Read the model definition and answer for the solid it produces. Units are mm, in the model's axes. Face numbers are marked on the shaded views. A direction names the side the tool comes from. Coordinates: 2 decimals unless noted, no trailing zeros. Loops run counter-clockwise (first coordinate to the right, second up) from the corner with the lowest first, then second, coordinate; pieces in that order, holes last.
from build123d import *

# Parameters (mm, degrees)
CROQUIS1_R              = 1.625
SALIENTE_EXTRUIR1_DEPTH = 3
CORTAR_EXTRUIR1_DEPTH   = 2
CROQUIS4_W              = 29.5
CROQUIS4_H              = 10.2
SALIENTE_EXTRUIR2_DEPTH = 3
SALIENTE_EXTRUIR3_DEPTH = 3
CROQUIS7_W              = 10
CROQUIS7_H              = 3
SALIENTE_EXTRUIR4_DEPTH = 5
CROQUIS9_W              = 10
CROQUIS9_H              = 3
SALIENTE_EXTRUIR5_DEPTH = 10
CROQUIS10_R             = 1.625
CORTAR_EXTRUIR2_DEPTH   = 3
CORTAR_EXTRUIR3_DEPTH   = 2


with BuildPart() as part:
    # Croquis1 → Saliente-Extruir1 (new body)
    with BuildSketch(Plane.XY):
        Polygon((-40.458841365, -24.7), (-77.458841365, -24.7), (-77.458841365, -14.45), (-47.958841365, -14.45), (-47.958841365, -17.2), (-40.458841365, -17.2), align=None)
        with Locations((-44.208841365, -20.95)):
            Circle(CROQUIS1_R, mode=Mode.SUBTRACT)
    extrude(amount=SALIENTE_EXTRUIR1_DEPTH)

    # Croquis2 → Cortar-Extruir1 (cut)
    with BuildSketch(Plane.XY.offset(3)):
        Polygon((-44.232492922, -17.739034302), (-46.977793452, -19.324034302), (-46.977793452, -22.494034302), (-44.232492922, -24.079034302), (-41.487192392, -22.494034302), (-41.487192392, -19.324034302), align=None)
    extrude(amount=-CORTAR_EXTRUIR1_DEPTH, mode=Mode.SUBTRACT)

    # Croquis4 → Saliente-Extruir2 (add)
    with BuildSketch(Plane(origin=(0, -14.45, 0), x_dir=(1, 0, 0), z_dir=(0, 1, 0))):
        with Locations((-62.708841365, 2.1)):
            Rectangle(CROQUIS4_W, CROQUIS4_H)
    extrude(amount=SALIENTE_EXTRUIR2_DEPTH)

    # Croquis6 → Saliente-Extruir3 (add)
    with BuildSketch(Plane.XY.offset(3)):
        Polygon((-62.708841365, -11.45), (-67.708841365, -11.45), (-67.708841365, -5), (-57.708841365, -5), (-57.708841365, -11.45), align=None)
    extrude(amount=-SALIENTE_EXTRUIR3_DEPTH)

    # Croquis7 → Saliente-Extruir4 (add)
    with BuildSketch(Plane(origin=(0, -5, 0), x_dir=(1, 0, 0), z_dir=(0, 1, 0))):
        with Locations((-62.708841365, -1.5)):
            Rectangle(CROQUIS7_W, CROQUIS7_H)
    extrude(amount=SALIENTE_EXTRUIR4_DEPTH)

    # Croquis9 → Saliente-Extruir5 (add)
    with BuildSketch(Plane.XY.offset(3)):
        with Locations((-62.708841365, -6.5)):
            Rectangle(CROQUIS9_W, CROQUIS9_H)
    extrude(amount=SALIENTE_EXTRUIR5_DEPTH)

    # Croquis10 → Cortar-Extruir2 (cut)
    with BuildSketch(Plane.XZ.offset(8)):
        with Locations(Location((-62.708841365, 8, 0), (0, 0, 270))):
            Circle(CROQUIS10_R)
    extrude(amount=-CORTAR_EXTRUIR2_DEPTH, mode=Mode.SUBTRACT)

    # Croquis11 → Cortar-Extruir3 (cut)
    with BuildSketch(Plane.XZ.offset(8)):
        Polygon((-62.708841365, 4.83), (-59.963540835, 6.415), (-59.963540835, 9.585), (-62.708841365, 11.17), (-65.454141895, 9.585), (-65.454141895, 6.415), align=None)
    extrude(amount=-CORTAR_EXTRUIR3_DEPTH, mode=Mode.SUBTRACT)


solid = part.part
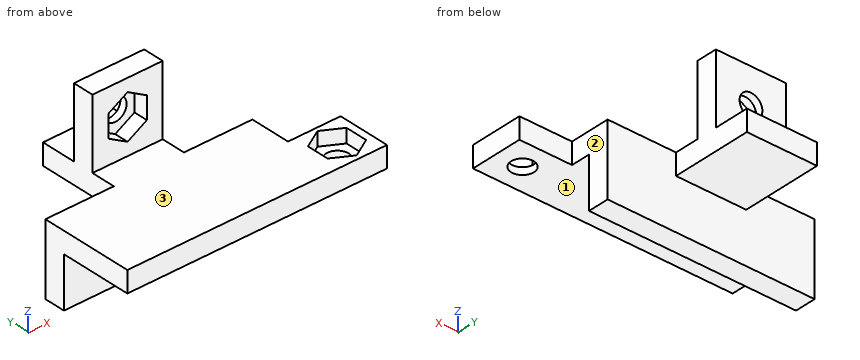
Item 1: Given pin 1 (5 mm diameter, centred on x = -63, y = -4.5, fed in from -Z); pin 2 (1 mm diameter, centred on y = -7, z = 8.5, fed in from +X); pin 3 (5 mm diameter, centred on x = -69.5, z = -3.5, fed in from +Y), each flat-ended and moving along its own axis, determine where each tip first touches the part or whether it passes through.
Numbers:
pin 1: stops at z = 0
pin 2: stops at x = -57.71
pin 3: stops at y = -11.45
Item 2: Find the intervals of material crossed by line 1 along X through (y, z) = (-5.7, 8); line 2 along X through (y, z) = (-20.95, 0.3); line 3 along Y through (x, z) = (-51, -3.75), in increasing order.
Numbers:
line 1: x = -67.71 to -64.33, -61.08 to -57.71
line 2: x = -77.46 to -45.83, -42.58 to -40.46
line 3: y = -14.45 to -11.45
Item 3: A cutting plane is placed at B-B on y = -20.95. Determine the outline of the cut face in (x, z).
Numbers:
outline: (-77.46, 0) - (-45.83, 0) - (-45.83, 1) - (-46.98, 1) - (-46.98, 3) - (-77.46, 3) - close; (-42.58, 0) - (-40.46, 0) - (-40.46, 3) - (-41.49, 3) - (-41.49, 1) - (-42.58, 1) - close
Item 4: Which of the six approach directions +Z, -Z, +X, -X, +Y, -Y give full straight-line access (tool end or side, diameter ignored) to the marked faces 1, 2 and 3?
Numbers:
face 1: -Z, +X, -X, -Y
face 2: +Z, -Z, +X, +Y
face 3: +Z, +X, -X, -Y
Item 5: A cutting plane is placed at C-C on x = -63.5. Determine the outline of the cut face in (y, z), then the cut area to 3 significant figures.
Numbers:
outline: (-24.7, 0) - (-14.45, 0) - (-14.45, -7.2) - (-11.45, -7.2) - (-11.45, 0) - (0, 0) - (0, 3) - (-5, 3) - (-5, 6.58) - (-6, 6.58) - (-6, 5.29) - (-8, 5.29) - (-8, 3) - (-24.7, 3) - close; (-8, 10.71) - (-6, 10.71) - (-6, 9.42) - (-5, 9.42) - (-5, 13) - (-8, 13) - close
area: 112 mm2
Item 6: A cutting plane is placed at A-A on z = 8. Determine the outline of the cut face in (x, y), then the cut area to 3 significant figures.
Numbers:
outline: (-67.71, -8) - (-65.45, -8) - (-65.45, -6) - (-64.33, -6) - (-64.33, -5) - (-67.71, -5) - close; (-61.08, -6) - (-59.96, -6) - (-59.96, -8) - (-57.71, -8) - (-57.71, -5) - (-61.08, -5) - close
area: 15.8 mm2
Item 7: A cutting plane is placed at D-D on z = -5. Determine the outline of the cut face in (x, y), then the cut area to 3 significant figures.
Numbers:
outline: (-77.46, -14.45) - (-47.96, -14.45) - (-47.96, -11.45) - (-77.46, -11.45) - close
area: 88.5 mm2
